```python
from build123d import *

# Parameters (mm, degrees)
F0_W     = 32.9
F0_H     = 22.2
F1_DEPTH = 10
F3_DEPTH = 25


with BuildPart() as f1:
    # F0 (on Top) → F1 (new body)
    with BuildSketch(Plane.XY):
        with Locations((16.45, -11.1)):
            Rectangle(F0_W, F0_H)
    extrude(amount=F1_DEPTH)

    # F2 (on face) → F3 (cut)
    with BuildSketch(Plane.XY.offset(10)):
        with BuildLine():
            Line((16.45, -11.1), (14.792127417, -9.981313941))
            ThreePointArc((14.792127417, -9.981313941), (14.45, -11.1), (14.792127417, -12.218686059))
            Line((14.792127417, -12.218686059), (16.45, -11.1))
        make_face()
        with BuildLine():
            ThreePointArc((18.107872583, -9.981313941), (16.45, -9.1), (14.792127417, -9.981313941))
            Line((14.792127417, -9.981313941), (16.45, -11.1))
            Line((16.45, -11.1), (18.107872583, -9.981313941))
        make_face()
        with BuildLine():
            Line((18.107872583, -12.218686059), (16.45, -11.1))
            Line((16.45, -11.1), (14.792127417, -12.218686059))
            ThreePointArc((14.792127417, -12.218686059), (16.45, -13.1), (18.107872583, -12.218686059))
        make_face()
        with BuildLine():
            Line((18.107872583, -9.981313941), (16.45, -11.1))
            Line((16.45, -11.1), (18.107872583, -12.218686059))
            ThreePointArc((18.107872583, -12.218686059), (18.3625565568, -11.6849165898), (18.45, -11.1))
            ThreePointArc((18.45, -11.1), (18.3625565568, -10.5150834102), (18.107872583, -9.981313941))
        make_face()
    extrude(amount=-F3_DEPTH, mode=Mode.SUBTRACT)


solid = f1.part
```
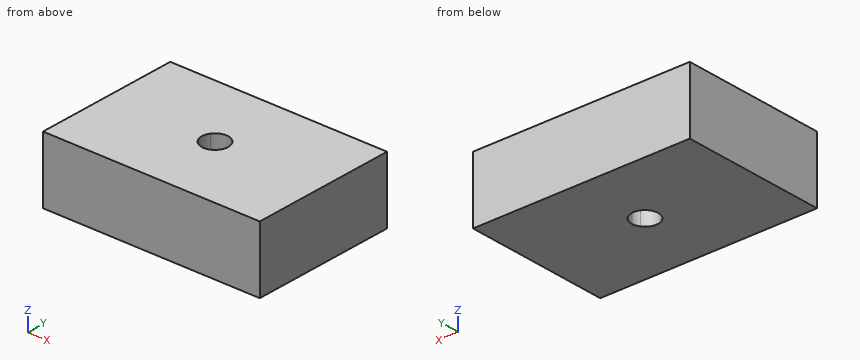
Read the model definition and answer for the solid it produces. Units are mm, in the model's axes. Coordinates: 2 decimals unless noted, no trailing zeros. Loops run counter-clockwise (first coordinate to the right, second up) from the corner with the lowest first, then second, coordinate; pieces in that order, holes last.
(1) The part is cut by section A-A (z = 6.25). Determine the outline of the cut face in (x, y).
Solution:
outline: (0, -22.2) - (32.9, -22.2) - (32.9, 0) - (0, 0) - close; hole circle Ø4 at (16.45, -11.1)
(2) Consider line 1 along X through (y, z) = (-9.5, 9.5); line 2 along X through (y, z) = (-10.25, 1.75); line 3 along Y through (x, z) = (15.5, 2). Determine where each line is inside the solid, lowest interval first.
Solution:
line 1: x = 0 to 15.25, 17.65 to 32.9
line 2: x = 0 to 14.64, 18.26 to 32.9
line 3: y = -22.2 to -12.86, -9.34 to 0
(3) A flat-ended cylindrical pin translates along its axis: pin 1 Ø4 at (x, z) = (19, 1.5) entering from +Y. Find the tip coordinate at first contact, or state that the pin passes through.
Solution:
pin 1: stops at y = 0
